```python
from build123d import *

# Parameters (mm, degrees)
F1_W     = 50.238024
F1_H     = 30.48
F2_DEPTH = 2.54
F3_DEPTH = 2.54
F4_W     = 2.54
F4_H     = 2.54
F5_DEPTH = 2.54
F6_W     = 2.54
F6_H     = 2.54
F7_DEPTH = 2.54


with BuildPart() as f2:
    # F1 (on Front) → F2 (new body)
    with BuildSketch(Plane.XZ):
        with Locations((7.288118, 12.7)):
            Rectangle(F1_W, F1_H)
    extrude(amount=-F2_DEPTH)

    # F0 (on Front) → F3 (cut, through all)
    with BuildSketch(Plane.XZ):
        Polygon((-8.940894, 25.4), (-15.290894, 25.4), (-2.829347, 0), (7.282625, 19.05), (13.632625, 19.05), (3.520653, 0), (9.870653, 0), (20.089414, 19.05), (26.439414, 19.05), (29.86713, 25.4), (3.759106, 25.4), (-2.829347, 13.97), align=None)
    extrude(amount=-F3_DEPTH, mode=Mode.SUBTRACT)

    # F4 (on face) → F5 (cut, through all)
    with BuildSketch(Plane.XZ):
        with Locations((31.13713, 7.62)):
            Rectangle(F4_W, F4_H)
        with Locations((31.13713, 1.27)):
            Rectangle(F4_W, F4_H)
    extrude(amount=-F5_DEPTH, mode=Mode.SUBTRACT)

    # F6 (on face) → F7 (join)
    with BuildSketch(Plane(origin=(-17.830894, 0, 0), x_dir=(0, -1, 0), z_dir=(-1, 0, 0))):
        with Locations((-1.27, 7.62)):
            Rectangle(F6_W, F6_H)
        with Locations((-1.27, 1.27)):
            Rectangle(F6_W, F6_H)
    extrude(amount=F7_DEPTH)


solid = f2.part
```
Work out the finished part from the listing and answer in its coordinate system (mm). A direction names the side the tool comes from. Coordinates: 2 decimals unless noted, no trailing zeros. Write each loop counter-clockwise with the first axis right and the second up, starting at its lowest first coordinate (ties: lowest second). Pieces come first, ordered by that corner, then holes.
Q1. A cutting plane is placed at A-A, the plane x = 23. Give the vertices of the cut face in (y, z), then the cut area to 3 significant figures.
Q2. Each of these flat-tipped pins is pushed along its axis until it touches: pin 1 Ø8 at (x, z) = (13.5, 20.5) entering from +Y; pin 2 Ø1.3 at (x, y) = (-19.5, 1.5) entering from -Z; pin 3 Ø0.8 at (x, y) = (-19, 1.5) entering from +Z; pin 4 Ø0.8 at (y, z) = (1.5, 1.5) entering from +X. Where does it stop, or does it pass through?
Q3. Find the intervals of material crossed by line 1 (Z direction, x = 30, y = 1.35); line 2 (X direction, y = 0.55, z = 8); line 3 (Z direction, x = 25, y = 1.15), in increasing order.
Q4. A cutting plane is placed at C-C, the plane z = 10. Give the vertices of the cut face in (x, y).
Q5. Determine the mould class of faces 6 (the face through (7, 1, -2.54)), 7 (the face through (-17.831, 1, -1)), 8 (the face through (28.13, 1.25, 22.18)), 9 (the face through (29.867, 1, 8)) for opening direction X: released by +X, released by -X, zero draft, split by the parting line, or undercut.
Q6. Which of the six approach directions +Z, -Z, +X, -X, +Y, -Y give full straight-line access (tool end or side, diameter ignored) to faces 1 (the face through (32.407, 1, 18)), 2 (the face through (-19, 1, 2.54)), 3 (the face through (23, 1, 19.05)), 4 (the face through (6, 2.54, 13)), 5 (the face through (29.867, 1, 1))?
Q7. A cutting plane is placed at D-D, the plane z = 17. Give the vertices of the cut face in (x, y), then the cut area to 3 significant figures.
Findings below:
1. outline: (0, -2.54) - (2.54, -2.54) - (2.54, 19.05) - (0, 19.05) - close; (0, 25.4) - (2.54, 25.4) - (2.54, 27.94) - (0, 27.94) - close
1. area: 61.3 mm2
2. pin 1: stops at y = 2.54
2. pin 2: stops at z = 0
2. pin 3: stops at z = 8.89
2. pin 4: stops at x = 29.87
3. line 1: z = -2.54 to 0, 2.54 to 6.35, 8.89 to 27.94
3. line 2: x = -20.37 to -6.75, 1.42 to 7.77, 14.16 to 29.87
3. line 3: z = -2.54 to 19.05, 25.4 to 27.94
4. outline: (-17.83, 0) - (-7.74, 0) - (-7.74, 2.54) - (-17.83, 2.54) - close; (2.48, 0) - (8.83, 0) - (8.83, 2.54) - (2.48, 2.54) - close; (15.23, 0) - (32.41, 0) - (32.41, 2.54) - (15.23, 2.54) - close
5. face 6: zero draft
5. face 7: released by -X
5. face 8: undercut
5. face 9: released by +X
6. face 1: +Z, -Z, +X, +Y, -Y
6. face 2: -X, +Y, -Y
6. face 3: +Y, -Y
6. face 4: +Z, -Z, +X, -X, +Y
6. face 5: +X, +Y, -Y
7. outline: (-17.83, 0) - (-11.17, 0) - (-11.17, 2.54) - (-17.83, 2.54) - close; (-4.45, 0) - (-1.08, 0) - (-1.08, 2.54) - (-4.45, 2.54) - close; (6.19, 0) - (12.54, 0) - (12.54, 2.54) - (6.19, 2.54) - close; (18.99, 0) - (32.41, 0) - (32.41, 2.54) - (18.99, 2.54) - close
7. area: 75.7 mm2
